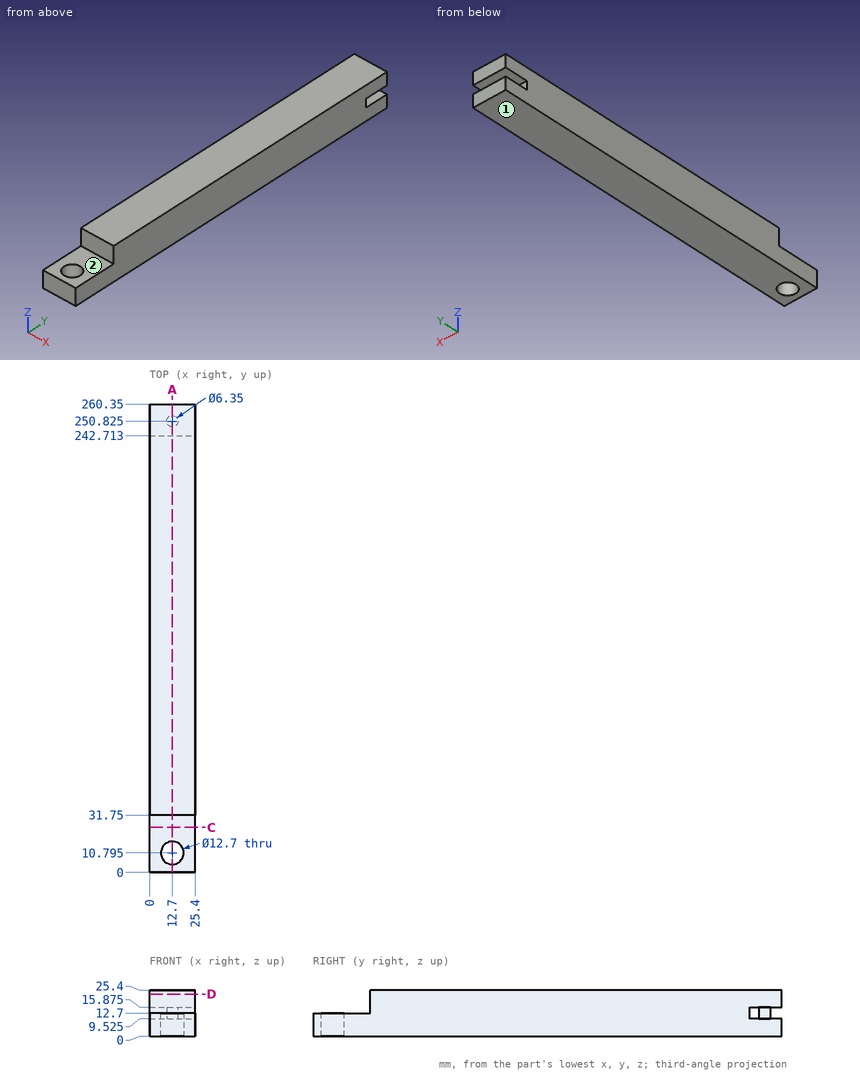
Part print with two shaded views. Sizes in mm from the minimum x, y, z corner. A direction names the side the tool comes from. Round coordinates to 2 decimals unless told otherwise and drop trailing zeros. Write each loop counter-clockwise with the first axis right and the second up, starting at its lowest first coordinate (ties: lowest second). Pieces come first, ordered by that corner, then holes. Notation, with made-up numbers: M 84.25,-28 L 143.25,-28 A23 ccw 143.25,10 Z; hole C -23.75,54 d9. An arc over 180 degrees is marked long. Answer as CSV lines item,"result". Start each with the question number.
1) Band-saw the part on D-D (z = 23.25). List the corners of the cut face in (x, y).
2) Band-saw the part on A-A (x = 12.7). Count the separate pieces of the cut face and the enclosed holes in it, then the cut area to 3 significant figures.
3) Drill centre lines: L1, parallel to Y at x = 19, z = 20.5; L2, parallel to Y at x = 17.75, z = 15; L3, parallel to Y at x = 16.5, z = 7. Where is each one in solid material? Low to high.
4) Which spindle directions (+Z, -Z, +X, -X, +Y, -Y) get a long thin tool onto all of the face, cutting with end or side? Do the marked faces 1 and 2. Say none if no direction does.
5) Drop flat-ended pins along their axis: pin 1 (14 mm diameter, centred on x = 15, z = 21.5, fed in from -Y); pin 2 (10 mm diameter, centred on x = 12.7, y = 10.795, fed in from +Z); pin 3 (1.5 mm diameter, centred on x = 15, z = 11, fed in from +Y); pin 4 (1 mm diameter, centred on x = 7, y = 47.5, fed in from -Z). Give the stop position or say it passes through.
6) Band-saw the part on C-C (y = 25). List the corners of the cut face in (x, z), then the cut area to 3 significant figures.
Worked out:
1,outline,"M 0,31.75 L 25.4,31.75 L 25.4,260.35 L 0,260.35 Z"
2,separate pieces,"2"
2,enclosed holes,"1"
2,area,"5,980 mm²"
3,L1,"31.75 to 260.35"
3,L2,"31.75 to 242.71"
3,L3,"0 to 5.71, 15.88 to 260.35"
4,face 1,"-Z, +X, -X, +Y, -Y"
4,face 2,"+Z, +X, -X, -Y"
5,pin 1,"y = 31.75"
5,pin 2,"through"
5,pin 3,"y = 253.6"
5,pin 4,"z = 0"
6,outline,"M 0,0 L 25.4,0 L 25.4,12.7 L 0,12.7 Z"
6,area,"323 mm²"
